Here's how the part is built. I have some questions about the finished solid (model axes, mm). A direction names the side the tool comes from. Round coordinates to 2 decimals unless told otherwise and drop trailing zeros. Loops run counter-clockwise (first coordinate to the right, second up) from the corner with the lowest first, then second, coordinate; pieces in that order, holes last. Notation, with made-up numbers: (24.25, 60) - (71.25, 60) arc R17 ccw to (71.25, 88) - close; hole circle Ø10 at (59, -25). An arc over 180 degrees is marked (long way). Return JSON: item names as keys, results as strings. Group by question number.
```python
from build123d import *

# Parameters (mm, degrees)
BOSS_EXTRUDE1_DEPTH = 20
SKETCH2_R           = 2.5
CUT_EXTRUDE1_DEPTH  = 56.518015094
FILLET1_R           = 10


with BuildPart() as part:
    # Sketch1 → Boss-Extrude1 (new body)
    with BuildSketch(Plane.XY):
        Polygon((-30, 13.5), (30, 13.5), (30, 1.5), (20, 1.5), (20, -13.5), (-20, -13.5), (-20, 1.5), (-30, 1.5), align=None)
    extrude(amount=BOSS_EXTRUDE1_DEPTH)

    # Sketch2 → Cut-Extrude1 (cut, through all)
    with BuildSketch(Plane(origin=(20, 0, 0), x_dir=(0, 0, -1), z_dir=(1, 0, 0))):
        with Locations(Location((-10, -6, 0), (0, 0, 90))):
            Circle(SKETCH2_R)
    extrude(amount=-CUT_EXTRUDE1_DEPTH, mode=Mode.SUBTRACT)

    # Fillet1
    fillet1_edges = [part.edges().sort_by_distance(p)[0] for p in [
        (0, -13.5, 0),
        (0, -13.5, 20),
    ]]
    fillet(fillet1_edges, radius=FILLET1_R - 0.0001)  # a hair under: the kernel refuses the full size


solid = part.part
```
Q1. Will these pins go through, and if not, where does the flat tip stop? pin 1 Ø3 at (x, y) = (0.5, 6.5) entering from -Z; pin 2 Ø6 at (y, z) = (-5.5, 9.5) entering from -X; pin 3 Ø4.5 at (y, z) = (-8, 5.5) entering from +X; pin 4 Ø1.5 at (x, z) = (9.5, 8.5) entering from -Y.
Q2. Imagine slicing it at D-D, the plane x = -21.5. List the corners of the cut face in (y, z) for me, and give its area (3 significant figures).
Q3. Imagine slicing it at C-C, the plane z = 2. List the corners of the cut face in (x, y) for me.
Q4. Imagine slicing it at B-B, the plane y = -6. List the corners of the cut face in (x, z) for me, and give its area (3 significant figures).
Q5. For faces 4 (the flat face through (-20, -3, 10)), 5 (the flat face through (30, 8, 10)), 6 (the flat face through (20, -4, 12)), which set-ups out of +Z, -Z, +X, -X, +Y, -Y let a thin tool reach every point of the face, with its end or its side?
Q6. Please list where these lines run through material, in increasing order: line 1 (X direction, y = -1.5, z = 11); line 2 (Y direction, x = 21, z = 2.5); line 3 (Z direction, x = 5.5, y = -6).
Q7. If we mould it in two halves opening along Z, with no side actions, what happens to faces 1 (the flat face through (0, 5, 0)), 2 (the cylindrical face through (0.28, -4.85, 7.78)), 3 (the flat face through (0, 5, 20))? For each: +Z half, -Z half, draft (parallel to the pull), parting line (faces both ways), or undercut.
Output values:
{
 "1": {"pin 1": "stops at z = 0", "pin 2": "stops at x = -20", "pin 3": "stops at x = 20", "pin 4": "stops at y = -13.47"},
 "2": {"outline": "(1.5, 0) - (13.5, 0) - (13.5, 20) - (1.5, 20) - close", "area": "240 mm^2"},
 "3": {"outline": "(-30, 1.5) - (-20, 1.5) - (-20, -9.5) - (20, -9.5) - (20, 1.5) - (30, 1.5) - (30, 13.5) - (-30, 13.5) - close"},
 "4": {"outline": "(-20, 0.32) - (20, 0.32) - (20, 7.5) - (-20, 7.5) - close; (-20, 12.5) - (20, 12.5) - (20, 19.68) - (-20, 19.68) - close", "area": "575 mm^2"},
 "5": {"face 4": "+Z, -Z, -X, -Y", "face 5": "+Z, -Z, +X, +Y, -Y", "face 6": "+Z, -Z, +X, -Y"},
 "6": {"line 1": "x = -20 to 20", "line 2": "y = 1.5 to 13.5", "line 3": "z = 0.32 to 7.5, 12.5 to 19.68"},
 "7": {"face 1": "-Z half", "face 2": "undercut", "face 3": "+Z half"}
}
